from build123d import *

# Parameters (mm, degrees)
SKETCH_1_W      = 14.591836735
SKETCH_1_H      = 24.132653061
EXTRUDE_1_DEPTH = 2
SKETCH_2_W      = 4.690013975
SKETCH_2_H      = 54.456273374
EXTRUDE_2_DEPTH = 16.5


with BuildPart() as part:
    # 草图1 → 凸台-拉伸1 (new body)
    with BuildSketch(Plane(origin=(0, 0, 0), x_dir=(1, 0, 0), z_dir=(0, 1, 0))):
        with BuildLine():
            Line((-23.5, -32.5), (23.5, -32.5))
            ThreePointArc((23.5, -32.5), (26.328427125, -31.328427125), (27.5, -28.5))
            Line((27.5, -28.5), (27.5, 28.5))
            ThreePointArc((27.5, 28.5), (26.328427125, 31.328427125), (23.5, 32.5))
            Line((23.5, 32.5), (-23.5, 32.5))
            ThreePointArc((-23.5, 32.5), (-26.328427125, 31.328427125), (-27.5, 28.5))
            Line((-27.5, 28.5), (-27.5, -28.5))
            ThreePointArc((-27.5, -28.5), (-26.328427125, -31.328427125), (-23.5, -32.5))
        make_face()
        with Locations((-7.295918368, -2.946428572)):
            Rectangle(SKETCH_1_W, SKETCH_1_H, mode=Mode.SUBTRACT)
    extrude(amount=EXTRUDE_1_DEPTH)

    # 草图2 → 凸台-拉伸2 (add)
    with BuildSketch(Plane.XZ):
        with Locations((-23.536921985, 0)):
            Rectangle(SKETCH_2_W, SKETCH_2_H)
    extrude(amount=EXTRUDE_2_DEPTH)


solid = part.part
For this review, take the finished solid that the model builds, in its own axes (mm). A direction names the side the tool comes from. Round coordinates to 2 decimals unless told otherwise and drop trailing zeros. Loops run counter-clockwise (first coordinate to the right, second up) from the corner with the lowest first, then second, coordinate; pieces in that order, holes last. Notation, with made-up numbers: (-17, 46.25) - (26, 46.25) arc R15 cw to (26, 50.25) - close; hole circle Ø6 at (-7.75, 12.5). An arc over 180 degrees is marked (long way). One line per item, written item: value. Start each with the question number.
Item 1: For faces 1 (the flat face through (-24, -8, 27.228)), 2 (the flat face through (-25.882, -8, 0)), 3 (the flat face through (0, 1, 3)), list the 3-axis set-ups (+Z, -Z, +X, -X, +Y, -Y) from which the entire face can be reached by the end or side of a thin tool; tool diameter is ignored.
Item 2: The part is to be moulded in two halves that separate along X. For faces 4 (the cylindrical face through (26.359, 0.986, -31.297)), 5 (the flat face through (-14.592, 1, 3)), 6 (the cylindrical face through (-26.359, 0.986, 31.297)), say which applies: +X half, -X half, draft (parallel to the pull), parting line (faces both ways), or undercut.
Item 3: Take a section at C-C (z = 22). Give the boundary of the cut face in (x, y).
Item 4: Take a section at A-A (z = 8.5). Give the boundary of the cut face in (x, y).
Item 5: Take a section at B-B (x = -8). Give the boundary of the cut face in (y, z), plus the area to 3 significant figures.
Item 6: Take a section at D-D (y = -6.25). Give the boundary of the cut face in (x, z), plus the area to 3 significant figures.
Item 7: For L1, parallel to Y at x = -23, z = -30; L2, parallel to X at y = -5.25, z = 8.5, list the stretches that pass through material, from the lowest coordinate up.
Item 8: Clearance check with flat-ended pins moving along their axes: pin 1 Ø1.4 at (x, y) = (-24, -10.5) entering from -Z; pin 2 Ø8 at (y, z) = (-10.5, 4.5) entering from -X; pin 3 Ø5 at (x, y) = (-23.5, -5.5) entering from +Z. State where each tip first meets the part, or that it passes through.
Answer below:
1. face 1: +Z, +X, -X, -Y
1. face 2: +Z, -Z, -X, -Y
1. face 3: +Y, -Y
2. face 4: +X half
2. face 5: undercut
2. face 6: -X half
3. outline: (-27.5, 0) - (-25.88, 0) - (-25.88, -16.5) - (-21.19, -16.5) - (-21.19, 0) - (27.5, 0) - (27.5, 2) - (-27.5, 2) - close
4. outline: (-27.5, 0) - (-25.88, 0) - (-25.88, -16.5) - (-21.19, -16.5) - (-21.19, 0) - (-14.59, 0) - (-14.59, 2) - (-27.5, 2) - close; (0, 0) - (27.5, 0) - (27.5, 2) - (0, 2) - close
5. outline: (0, -32.5) - (2, -32.5) - (2, -9.12) - (0, -9.12) - close; (0, 15.01) - (2, 15.01) - (2, 32.5) - (0, 32.5) - close
5. area: 81.7 mm2
6. outline: (-25.88, -27.23) - (-21.19, -27.23) - (-21.19, 27.23) - (-25.88, 27.23) - close
6. area: 255 mm2
7. L1: y = 0 to 2
7. L2: x = -25.88 to -21.19
8. pin 1: stops at z = -27.23
8. pin 2: stops at x = -25.88
8. pin 3: stops at z = 27.23
